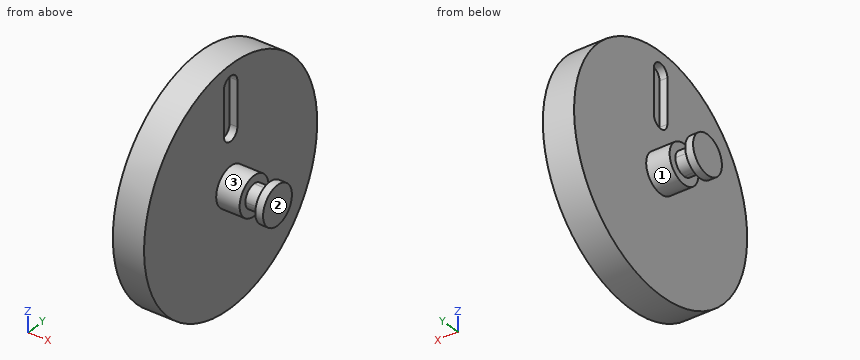
```python
from build123d import *

# Parameters (mm, degrees)
SKETCH_1_R          = 75
EXTRUDE_1_DEPTH     = 10
SKETCH_2_R          = 12.5
EXTRUDE_2_DEPTH     = 30
SKETCH_3_W          = 10
SKETCH_3_H          = 5
CUT_EXTRUDE_1_DEPTH = 5


with BuildPart() as part:
    # 草图1 → 凸台-拉伸1 (new body)
    with BuildSketch(Plane(origin=(0, 0, 0), x_dir=(0, 0, -1), z_dir=(1, 0, 0))):
        Circle(SKETCH_1_R)
    extrude_1 = extrude(amount=EXTRUDE_1_DEPTH)

    # 草图2 → 凸台-拉伸2 (add)
    with BuildSketch(Plane(origin=(10, 0, 0), x_dir=(0, 0, -1), z_dir=(1, 0, 0))):
        Circle(SKETCH_2_R)
    extrude_2 = extrude(amount=EXTRUDE_2_DEPTH)

    # 镜向1: 凸台-拉伸1, 凸台-拉伸2 across plane
    add(extrude_1.mirror(Plane(origin=(0, 0, 0), x_dir=(0, 0, 1), z_dir=(1, 0, 0))))
    add(extrude_2.mirror(Plane(origin=(0, 0, 0), x_dir=(0, 0, 1), z_dir=(1, 0, 0))))

    # 切除-扫描1: sweep along a curve in space
    with BuildLine() as sweep_1_path:
        ThreePointArc((-40, 0, -12.5), (-40, 8.838834765, -8.838834765), (-40, 12.5, 0))
        ThreePointArc((-40, 12.5, 0), (-40, 8.838834765, 8.838834765), (-40, 0, 12.5))
        ThreePointArc((-40, 0, 12.5), (-40, -8.838834765, 8.838834765), (-40, -12.5, 0))
        ThreePointArc((-40, -12.5, 0), (-40, -8.838834765, -8.838834765), (-40, 0, -12.5))
    # 草图3 → 切除-扫描1 (sweep, cut)
    with BuildSketch(Plane(origin=(0, 0, 0), x_dir=(1, 0, 0), z_dir=(0, 1, 0))):
        with Locations((-30, 10)):
            Rectangle(SKETCH_3_W, SKETCH_3_H)
    sweep_1 = sweep(path=sweep_1_path.line, mode=Mode.SUBTRACT)

    # 镜向2: 切除-扫描1 across plane
    add(sweep_1.mirror(Plane(origin=(0, 0, 0), x_dir=(0, 0, 1), z_dir=(1, 0, 0))), mode=Mode.SUBTRACT)

    # 草图5 → 切除-拉伸1 (cut)
    with BuildSketch(Plane.ZY.offset(10)):
        with BuildLine():
            Line((62.177784285, -5.817003296), (33.496104549, -5.817003296))
            ThreePointArc((33.496104549, -5.817003296), (27.679101253, 0), (33.496104549, 5.817003296))
            Line((33.496104549, 5.817003296), (62.177784285, 5.817003296))
            ThreePointArc((62.177784285, 5.817003296), (67.994787582, 0), (62.177784285, -5.817003296))
        make_face()
    cut_extrude_1 = extrude(amount=-CUT_EXTRUDE_1_DEPTH, mode=Mode.SUBTRACT)

    # 镜向3: 切除-拉伸1 across plane
    add(cut_extrude_1.mirror(Plane(origin=(0, 0, 0), x_dir=(0, 0, 1), z_dir=(1, 0, 0))), mode=Mode.SUBTRACT)


solid = part.part
```
For this review, take the finished solid that the model builds, in its own axes (mm). Face numbers are marked on the shaded views. A direction names the side the tool comes from. Coordinates: 2 decimals unless noted, no trailing zeros. Order: outer loops, then holes, each group sorted by start corner. A loop starts at its lowest first (then second) coordinate and runs counter-clockwise, first axis right, second up. Notation, with made-up numbers: (-33, 71.25) -> (23, 71.25) arc R6 ccw to (23, 76.25) -> close; hole circle Ø5 at (48.5, 66.25). An arc over 180 degrees is marked (long way). Answer as CSV lines item,"result".
Q1. For the marked faces 1, 2 and 3, list the 3-axis set-ups (+Z, -Z, +X, -X, +Y, -Y) from which the entire face can be reached by the end or side of a thin tool; tool diameter is ignored.
Model answer:
face 1,"-X"
face 2,"+Z, -Z, +X, +Y, -Y"
face 3,"+X"
Q2. We need section C-C (y = 29.5). State the section outline as (x, z) points, plus the area to 3 significant figures.
Model answer:
outline,"(-10, -68.95) -> (10, -68.95) -> (10, 68.95) -> (-10, 68.95) -> close"
area,"2,760 mm2"
Q3. We need section A-A (x = 14). State the section outline as (y, z) points.
Model answer:
outline,"circle Ø25 at (0, 0)"
Q4. Wall thickness on line 1 along X through (y, z) = (-48, -4.5); line 2 along Z through (x, y) = (31.5, 0.5); line 3 along Y through (x, z) = (4, -1): over which ranges is each line inside the solid? List them lowest first. Write a range as [from, to].
Model answer:
line 1,"x = [-10, 10]"
line 2,"z = [-7.48, 7.48]"
line 3,"y = [-74.99, 74.99]"
Q5. We need section B-B (z = 24). State the section outline as (x, y) points, plus the area to 3 significant figures.
Model answer:
outline,"(-10, -71.06) -> (10, -71.06) -> (10, 71.06) -> (-10, 71.06) -> close"
area,"2,840 mm2"
Q6. Clearance check with flat-ended pins moving along their axes: pin 1 Ø9.5 at (y, z) = (1, 42) entering from +X; pin 2 Ø5 at (x, y) = (-5.5, 7) entering from +Z; pin 3 Ø5.5 at (x, z) = (-7, 41) entering from -Y. State where each tip first meets the part, or that it passes through.
Model answer:
pin 1,"stops at x = 5"
pin 2,"stops at z = 74.86"
pin 3,"stops at y = -64.51"
